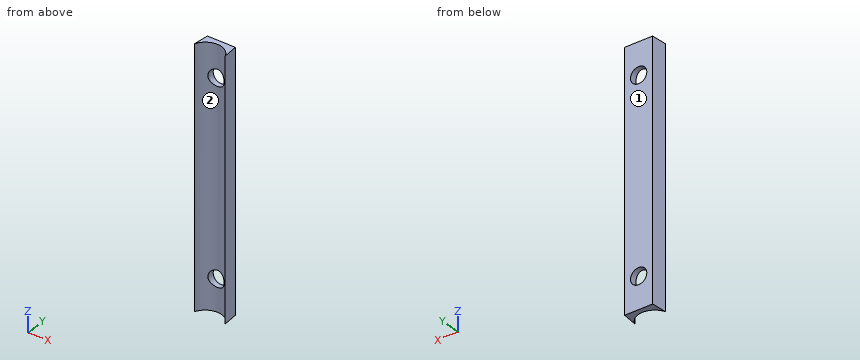
from build123d import *

# Parameters (mm, degrees)
CYLINDER001_R          = 3.2
CYLINDER001_DEPTH      = 10
CYLINDER001_ROLL_ANGLE = 90
CYLINDER_R             = 3.2
CYLINDER_DEPTH         = 10
CYLINDER_ROLL_ANGLE    = 90
PAD_DEPTH              = 50


with BuildPart() as cylinder001:
    # Cylinder001 → Cylinder001 (new body)
    with BuildSketch(Plane.XY):
        Circle(CYLINDER001_R)
    extrude(amount=CYLINDER001_DEPTH)


with BuildPart() as cylinder001_1:
    # Cylinder001 roll: moved
    add(cylinder001.part.rotate(Axis((0, 0, 0), (1, 0, 0)), CYLINDER001_ROLL_ANGLE))


with BuildPart() as cylinder001_2:
    # Cylinder001 placement: moved
    add(cylinder001_1.part.moved(Location((0, 2, -37.5))))


with BuildPart() as cylinder:
    # Cylinder → Cylinder (new body)
    with BuildSketch(Plane.XY):
        Circle(CYLINDER_R)
    extrude(amount=CYLINDER_DEPTH)


with BuildPart() as cylinder_1:
    # Cylinder roll: moved
    add(cylinder.part.rotate(Axis((0, 0, 0), (1, 0, 0)), CYLINDER_ROLL_ANGLE))


with BuildPart() as cylinder_2:
    # Cylinder placement: moved
    add(cylinder_1.part.moved(Location((0, 2, 37.5))))


with BuildPart() as cut001:
    # Sketch001 → Pad (new body, symmetric)
    with BuildSketch(Plane.XY):
        with BuildLine():
            ThreePointArc((6, -5.97913), (0, -1.97913), (-6, -5.97913))
            Line((-5.5, 0), (-6, -5.97913))
            Line((-5.5, 0), (5.5, 0))
            Line((5.5, 0), (6, -5.97913))
        make_face()
    extrude(amount=PAD_DEPTH, both=True)

    # Cut: cut Cylinder
    add(cylinder_2.part, mode=Mode.SUBTRACT)

    # Cut001: cut Cylinder001
    add(cylinder001_2.part, mode=Mode.SUBTRACT)


solid = cut001.part
Could you check a few things on this model? Use its own coordinates, in mm. Face numbers are marked on the shaded views. Give positions to 0.01 mm unless a question says otherwise; leave off trailing zeros. Order: outer loops, then holes, each group sorted by start corner. A loop starts at its lowest first (then second) coordinate and runs counter-clockwise, first axis right, second up.
Item 1: If we section it at D-D, the plane z = 19: Write out the boundary of the cut face in (x, y), plus the area to 3 significant figures.
Item 2: If we section it at A-A, the plane z = -37.5: Write out the boundary of the cut face in (x, y), plus the area to 3 significant figures.
Item 3: I need wall thicknesses on line 1 (Z direction, x = 0, y = -1.1); line 2 (Z direction, x = -1.5, y = -1.45); line 3 (X direction, y = -3.85, z = 24). Which ranges of each line are inside material? Lowest first, please.
Item 4: If we section it at B-B, the plane x = 0: Write out the boundary of the cut face in (y, z).
Item 5: If we mould it in two halves opening along X, with no side actions, what happens to the marked faces 1 and 2? For each: pulls with the +X half, pulls with the -X half, needs draft (parallel to the pull), parting line crosses it, or undercut.
Item 6: If we section it at C-C, the plane y = -4.8: Write out the boundary of the cut face in (x, z).
Item 7: I'm going to push flat-ended pins straight in: pin 1 (1.5 mm diameter, centred on y = -2.5, z = -7, fed in from -X); pin 2 (2 mm diameter, centred on x = -4.5, z = -18, fed in from -Y) (3 decimals). Where does each tip first touch, or does it pass through?
Values:
1. outline: (-6, -5.98) arc R6.5 cw to (6, -5.98) - (5.5, 0) - (-5.5, 0) - close
1. area: 34.1 mm2
2. outline: (-6, -5.98) arc R6.5 cw to (-3.2, -2.82) - (-3.2, 0) - (-5.5, 0) - close; (3.2, -2.82) arc R6.5 cw to (6, -5.98) - (5.5, 0) - (3.2, 0) - close
2. area: 19.7 mm2
3. line 1: z = -50 to -40.7, -34.3 to 34.3, 40.7 to 50
3. line 2: z = -50 to -40.33, -34.67 to 34.67, 40.33 to 50
3. line 3: x = -5.82 to -4.56, 4.56 to 5.82
4. outline: (-1.98, -50) - (0, -50) - (0, -40.7) - (-1.98, -40.7) - close; (-1.98, -34.3) - (0, -34.3) - (0, 34.3) - (-1.98, 34.3) - close; (-1.98, 40.7) - (0, 40.7) - (0, 50) - (-1.98, 50) - close
5. face 1: needs draft
5. face 2: undercut
6. outline: (-5.9, -50) - (-5.36, -50) - (-5.36, 50) - (-5.9, 50) - close; (5.36, -50) - (5.9, -50) - (5.9, 50) - (5.36, 50) - close
7. pin 1: stops at x = -5.77
7. pin 2: stops at y = -5.015
